Could you check a few things on this model? Use its own coordinates, in mm. Coordinates: 2 decimals unless noted, no trailing zeros. Loops run counter-clockwise (first coordinate to the right, second up) from the corner with the lowest first, then second, coordinate; pieces in that order, holes last.
from build123d import *

# Parameters (mm, degrees)
ESQUISSE1_W                         = 160
ESQUISSE1_H                         = 100
BOSS_EXTRU_1_DEPTH                  = 2
ENL_V_MAT_EXTRU_1_DEPTH             = 2
ENL_V_MAT_EXTRU_2_DEPTH             = 2
D_GAGEMENT_M21_D                    = 2.4
D_GAGEMENT_M21_DEPTH                = 2.001
D_GAGEMENT_M22_D                    = 2.4
D_GAGEMENT_M22_DEPTH                = 2.001
ENL_V_MAT_EXTRU_5_REACH             = 4
ESQUISSE11_W                        = 8
ESQUISSE11_H                        = 68
ENL_V_MAT_EXTRU_5_DIRECTION_2_DEPTH = 1


with BuildPart() as part:
    # Esquisse1 → Boss.-Extru.1 (new body)
    with BuildSketch(Plane(origin=(0, 0, 0), x_dir=(1, 0, 0), z_dir=(0, 1, 0))):
        with Locations((80, 50)):
            Rectangle(ESQUISSE1_W, ESQUISSE1_H)
    extrude(amount=BOSS_EXTRU_1_DEPTH)

    # Esquisse2 → Enlèv. mat.-Extru.1 (cut)
    with BuildSketch(Plane(origin=(0, 2, 0), x_dir=(1, 0, 0), z_dir=(0, 1, 0))):
        Polygon((30, 0), (0, 30), (0, 0), align=None)
        Polygon((30, 100), (0, 70), (0, 100), align=None)
        Polygon((130, 0), (160, 30), (160, 0), align=None)
        Polygon((130, 100), (160, 100), (160, 70), align=None)
    extrude(amount=-ENL_V_MAT_EXTRU_1_DEPTH, mode=Mode.SUBTRACT)

    # Esquisse3 → Enlèv. mat.-Extru.2 (cut)
    with BuildSketch(Plane(origin=(0, 2, 0), x_dir=(1, 0, 0), z_dir=(0, 1, 0))):
        with BuildLine():
            Line((65.05, 43), (65.05, 33))
            ThreePointArc((65.05, 33), (64, 31.95), (62.95, 33))
            Line((62.95, 33), (62.95, 43))
            ThreePointArc((62.95, 43), (64, 44.05), (65.05, 43))
        make_face()
        with BuildLine():
            Line((50.95, 33), (50.95, 43))
            ThreePointArc((50.95, 43), (52, 44.05), (53.05, 43))
            Line((53.05, 43), (53.05, 33))
            ThreePointArc((53.05, 33), (52, 31.95), (50.95, 33))
        make_face()
        with BuildLine():
            Line((109.05, 33), (109.05, 43))
            ThreePointArc((109.05, 43), (108, 44.05), (106.95, 43))
            Line((106.95, 43), (106.95, 33))
            ThreePointArc((106.95, 33), (108, 31.95), (109.05, 33))
        make_face()
        with BuildLine():
            Line((94.95, 43), (94.95, 33))
            ThreePointArc((94.95, 33), (96, 31.95), (97.05, 33))
            Line((97.05, 33), (97.05, 43))
            ThreePointArc((97.05, 43), (96, 44.05), (94.95, 43))
        make_face()
        with BuildLine():
            Line((50.95, 67), (50.95, 57))
            ThreePointArc((50.95, 57), (52, 55.95), (53.05, 57))
            Line((53.05, 57), (53.05, 67))
            ThreePointArc((53.05, 67), (52, 68.05), (50.95, 67))
        make_face()
        with BuildLine():
            Line((65.05, 57), (65.05, 67))
            ThreePointArc((65.05, 67), (64, 68.05), (62.95, 67))
            Line((62.95, 67), (62.95, 57))
            ThreePointArc((62.95, 57), (64, 55.95), (65.05, 57))
        make_face()
        with BuildLine():
            Line((94.95, 57), (94.95, 67))
            ThreePointArc((94.95, 67), (96, 68.05), (97.05, 67))
            Line((97.05, 67), (97.05, 57))
            ThreePointArc((97.05, 57), (96, 55.95), (94.95, 57))
        make_face()
        with BuildLine():
            Line((109.05, 67), (109.05, 57))
            ThreePointArc((109.05, 57), (108, 55.95), (106.95, 57))
            Line((106.95, 57), (106.95, 67))
            ThreePointArc((106.95, 67), (108, 68.05), (109.05, 67))
        make_face()
    extrude(amount=-ENL_V_MAT_EXTRU_2_DEPTH, mode=Mode.SUBTRACT)

    # Dégagement M21
    with Locations(Plane(origin=(0, 2, 0), x_dir=(1, 0, 0), z_dir=(0, 1, 0))):
        with Locations((28, 39), (28, 61), (7, 61), (7, 39)):
            d_gagement_m21 = Hole(D_GAGEMENT_M21_D / 2, depth=D_GAGEMENT_M21_DEPTH)

    # Dégagement M22
    with Locations(Plane(origin=(0, 2, 0), x_dir=(1, 0, 0), z_dir=(0, 1, 0))):
        with Locations((58, 14), (58, 86)):
            d_gagement_m22 = Hole(D_GAGEMENT_M22_D / 2, depth=D_GAGEMENT_M22_DEPTH)

    # Symétrie1: Dégagement M21, Dégagement M22 across plane
    add(d_gagement_m21.mirror(Plane.ZY.offset(-80)), mode=Mode.SUBTRACT)
    add(d_gagement_m22.mirror(Plane.ZY.offset(-80)), mode=Mode.SUBTRACT)

    # Esquisse11 → Enlèv. mat.-Extru.5 (cut, up to next)
    with BuildSketch(Plane(origin=(0, 2, 0), x_dir=(1, 0, 0), z_dir=(0, 1, 0)), mode=Mode.PRIVATE) as enl_v_mat_extru_5_sk1:
        with Locations((35.5, 50)):
            Rectangle(ESQUISSE11_W, ESQUISSE11_H)
    enl_v_mat_extru_5_tool1 = extrude(enl_v_mat_extru_5_sk1.sketch, amount=-ENL_V_MAT_EXTRU_5_REACH, mode=Mode.PRIVATE) & part.part
    add(enl_v_mat_extru_5_tool1.solids().sort_by_distance((35.5, 2, -50))[0], mode=Mode.SUBTRACT)
    # Esquisse11 → Enlèv. mat.-Extru.5 (cut, up to next)
    with BuildSketch(Plane(origin=(0, 2, 0), x_dir=(1, 0, 0), z_dir=(0, 1, 0)), mode=Mode.PRIVATE) as enl_v_mat_extru_5_sk2:
        with Locations((124.5, 50)):
            Rectangle(ESQUISSE11_W, ESQUISSE11_H)
    enl_v_mat_extru_5_tool2 = extrude(enl_v_mat_extru_5_sk2.sketch, amount=-ENL_V_MAT_EXTRU_5_REACH, mode=Mode.PRIVATE) & part.part
    add(enl_v_mat_extru_5_tool2.solids().sort_by_distance((124.5, 2, -50))[0], mode=Mode.SUBTRACT)

    # Esquisse11 → Enlèv. mat.-Extru.5 direction 2 (cut)
    with BuildSketch(Plane(origin=(0, 2, 0), x_dir=(1, 0, 0), z_dir=(0, 1, 0))):
        with Locations((35.5, 50)):
            Rectangle(ESQUISSE11_W, ESQUISSE11_H)
        with Locations((124.5, 50)):
            Rectangle(ESQUISSE11_W, ESQUISSE11_H)
    extrude(amount=ENL_V_MAT_EXTRU_5_DIRECTION_2_DEPTH, mode=Mode.SUBTRACT)


solid = part.part
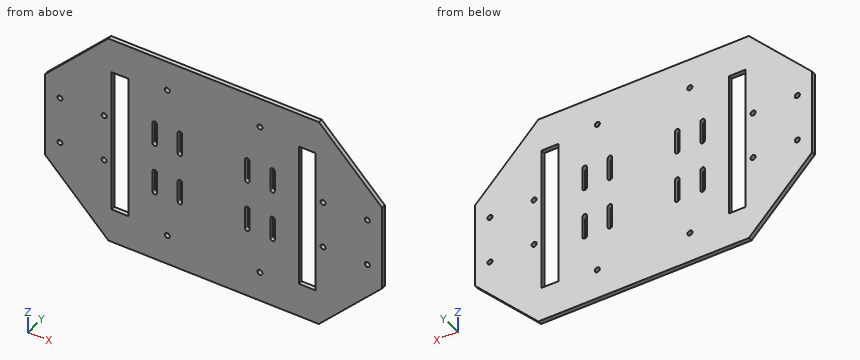
(1) I need wall thicknesses on probe 1 along Z at (x, y) = (58, 1.15); probe 2 along X at (y, z) = (1.8, -74.5); probe 3 along X at (y, z) = (0.9, -69). Which ranges of each line are inside material? Lowest first, please.
Answers:
probe 1: z = -100 to -87.2, -84.8 to -15.2, -12.8 to 0
probe 2: x = 4.5 to 31.5, 39.5 to 120.5, 128.5 to 155.5
probe 3: x = 0 to 31.5, 39.5 to 120.5, 128.5 to 160
(2) Imagine slicing it at B-B, the plane y = 1.5. State how many separate pieces and enclosed holes the cut face has, and give its area (3 significant figures).
Answers:
separate pieces: 1
enclosed holes: 22
area: 12,900 mm2
(3) Imagine slicing it at A-A, the plane z = -82. Write out the boundary of the cut face in (x, y), and give its area (3 significant figures).
Answers:
outline: (12, 0) - (31.5, 0) - (31.5, 2) - (12, 2) - close; (39.5, 0) - (120.5, 0) - (120.5, 2) - (39.5, 2) - close; (128.5, 0) - (148, 0) - (148, 2) - (128.5, 2) - close
area: 240 mm2
(4) For pin 1 (0.6 mm diameter, centred on y = 1.5, z = -38.5, fed in from -X), with a flat end and sliding along its axis, tell me the tip position at first contact or that it passes through.
Answers:
pin 1: stops at x = 0
